Model file for the job. Use its own axes, mm. A direction names the side the tool comes from. Round coordinates to 2 decimals unless told otherwise and drop trailing zeros. Order: outer loops, then holes, each group sorted by start corner. A loop starts at its lowest first (then second) coordinate and runs counter-clockwise, first axis right, second up. Notation, with made-up numbers: (-1, 12.5) -> (30, 12.5) arc R6 cw to (30, 21.5) -> close; hole circle Ø8 at (81.5, -35.75). An arc over 180 degrees is marked (long way). Answer as CSV lines item,"result".
Autodesk Inventor part; units mm, degrees
ref_plane "YZ Plane" through (0, 0, 0) normal (1, 0, 0) x (0, 1, 0)
ref_plane "XZ Plane" through (0, 0, 0) normal (0, 1, 0) x (-1, 0, 0)
ref_plane "XY Plane" through (0, 0, 0) normal (0, 0, 1) x (1, 0, 0)
sketch "Sketch1" plane through (0, 0, 0) normal (0, 0, 1) x (1, 0, 0)
  line L0 (0, -46.3) -> (0, 3)
  line L1 (3, 3) -> (43, 3)
  line L2 (3, 3) -> (0, 3)
  line L3 (43, 0) -> (43, 3)
  line L4 (43, 1.7) -> (86, 1.7)
  line L5 (86, -1.3) -> (86, 1.7)
  line L6 (86, -1.3) -> (86, -46.3)
  line L7 (86, -46.3) -> (86, -49.3)
  line L8 (86, -49.3) -> (0, -49.3)
  line L9 (0, -46.3) -> (0, -49.3)
  line L10 (3, -46.3) -> (0, -46.3)
  line L11 (3, 3) -> (3, 0)
  line L12 (43, -1.3) -> (43, 1.7)
  line L13 (83, -46.3) -> (83, -1.3)
  line L14 (83, -46.3) -> (86, -46.3)
  line L15 (86, -1.3) -> (86, -46.3)
  line L16 (83, -1.3) -> (86, -1.3)
  line L17 (83, -46.3) -> (76, -46.3)
  line L18 (76, -46.3) -> (76, -49.3)
  line L19 (83, -1.3) -> (76, -1.3)
  line L20 (76, -1.3) -> (76, 1.7)
  line L21 (43, -1.3) -> (48, -1.3)
  line L22 (48, -1.3) -> (48, 1.7)
  line L23 (43, 0) -> (38, 0)
  line L24 (38, 0) -> (38, 3)
  line L25 (3, -46.3) -> (10, -46.3)
  line L26 (10, -46.3) -> (10, -49.3)
  line L27 (3, 0) -> (3, -7)
  line L28 (3, -7) -> (0, -7)
  line L29 (13.777, 0) -> (8.777, 0)
  line L30 (8.777, 0) -> (8.777, 3)
  line L31 (8.777, 3) -> (13.777, 3)
  line L32 (13.777, 3) -> (13.777, 0)
  line L33 (48, -49.3) -> (38, -49.3)
  line L34 (38, -49.3) -> (38, -46.3)
  line L35 (38, -46.3) -> (48, -46.3)
  line L36 (48, -46.3) -> (48, -49.3)
  line L37 (86, -6.3) -> (83, -6.3)
  line L38 (83, -41.3) -> (86, -41.3)
  point P0 (0, 0)
  point P1 (43, -49.3)
  dimension "d0" = 10
  dimension "d1" = 10
  dimension "d2" = 10
  dimension "d3" = 10
  dimension "d4" = 10
  dimension "d5" = 5
  dimension "d6" = 5
  dimension "d7" = 5
  dimension "d10" = 5
  dimension "d11" = 5
extrude "Extrusion1" add sketch "Sketch1" along normal blind 3 contours L0 L28 L27 L11 L1 L30 L29 L32 L24 L23 L12 L21 L22 L4 L20 L19 L13 L17 L18 L8 L36 L35 L34 L26 L25 L10 | L38 L13 L37 L6
properties part number "top" material "Acrylic, Clear"
Q1. Flat gauge pins, fed straight in: pin 1 (0.9 mm diameter, centred on x = 2, z = 2, fed in from +Y); pin 2 (6 mm diameter, centred on x = 76.5, y = -22.5, fed in from -Z); pin 3 (1 mm diameter, centred on y = -1, z = 2, fed in from +X); pin 4 (1.5 mm diameter, centred on y = -48, z = 1.5, fed in from -X). Where does each tip first touch, or does it go through?
Checks:
pin 1,"y = -7"
pin 2,"z = 0"
pin 3,"x = 83"
pin 4,"x = 10"
Q2. Wall check: L1, parallel to Y at x = 82, z = 0.8; L2, parallel to Y at x = 64.5, z = 2.15; L3, parallel to X at y = -6, z = 0.5. Give the ranges that are in metal, low to high. Write a range as [from, to].
Checks:
L1,"[-46.3, -1.3]"
L2,"[-49.3, 1.7]"
L3,"[3, 83]"
Q3. Saw through at C-C (x = 6). Write the cut outline in (y, z).
Checks:
outline,"(-46.3, 0) -> (3, 0) -> (3, 3) -> (-46.3, 3) -> close"
Q4. Saw through at B-B (y = -45). Write the cut outline in (x, z).
Checks:
outline,"(0, 0) -> (83, 0) -> (83, 3) -> (0, 3) -> close"
Q5. Tool access for faces 4 (the flat face through (83, -44, 1)), 5 (the flat face through (80, -1.3, 1)), 6 (the flat face through (13.777, 2, 1)), 7 (the flat face through (48, -48, 1)), 8 (the flat face through (2, -7, 1)): list every direction of +Z, -Z, +X, -X, +Y, -Y with a clear straight run to the whole face (end or side of a thin tool).
Checks:
face 4,"+Z, -Z, +X, -Y"
face 5,"+Z, -Z, +X, +Y"
face 6,"+Z, -Z, +Y"
face 7,"+Z, -Z, -Y"
face 8,"+Z, -Z, -X, +Y"
Q6. Mould opens along X. For faces 1 (the flat face through (38, -48, 1)), 2 (the flat face through (5, -46.3, 1)), 3 (the flat face through (10, -48, 1)) say: +X half, -X half, draft (parallel to the pull), parting line (faces both ways), or undercut.
Checks:
face 1,"undercut"
face 2,"draft"
face 3,"-X half"
